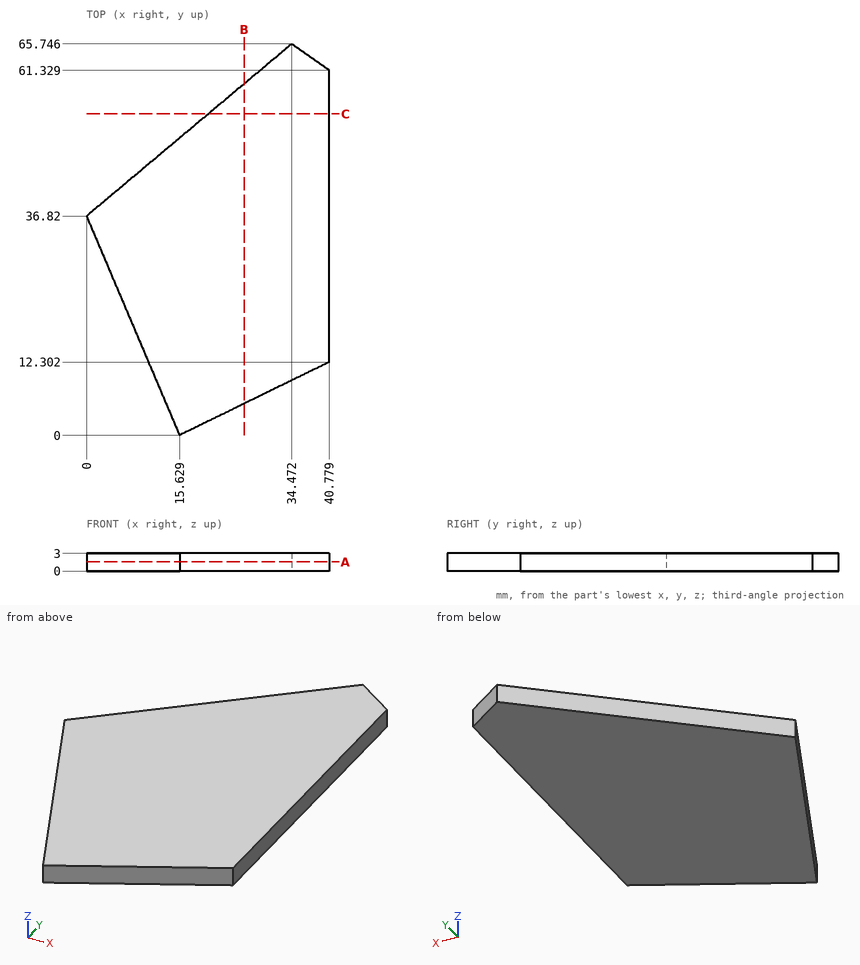
Source: three-view drawing plus pictorial views. Frame: mm from the lowest corner of the part. Round coordinates to 2 decimals unless told otherwise and drop trailing zeros. Loops run counter-clockwise (first coordinate to the right, second up) from the corner with the lowest first, then second, coordinate; pieces in that order, holes last. Notation, with made-up numbers: M -5.5,67.5 L 17.5,67.5 A4 cw 17.5,71.5 Z; hole C 86,73 d6. An arc over 180 degrees is marked long. Put each result on its own line as item: value. Start each with the question number.
(1) Contact query for a flat-ended pin moving along its axis: pin 1 Ø8 at (x, y) = (9.5, 22) entering from -Z. Output: stop coordinate, or through.
(2) Section query A-A (z = 1.55). Return loops of the section in (x, y) (1 decimal), then the cut area to 3 significant figures.
(3) Material intervals for line 1 along X through (y, z) = (27, 0.65); line 2 along Y through (x, z) = (23, 1.5) (1 decimal); line 3 along Y through (x, z) = (9.5, 1.85) (1 decimal), sorted ascending. Write a range as [from, to].
(4) Section query C-C (y = 54). Return loops of the section in (x, z) (1 decimal).
(5) Section query B-B (x = 26.5). Return loops of the section in (y, z), then the cut area to 3 significant figures.
Findings below:
1. pin 1: stops at z = 0
2. outline: M 0,36.8 L 15.6,0 L 40.8,12.3 L 40.8,61.3 L 34.5,65.7 Z
2. area: 1,730 mm2
3. line 1: x = [4.17, 40.78]
3. line 2: y = [3.6, 56.1]
3. line 3: y = [14.4, 44.8]
4. outline: M 20.5,0 L 40.8,0 L 40.8,3 L 20.5,3 Z
5. outline: M 5.32,0 L 59.06,0 L 59.06,3 L 5.32,3 Z
5. area: 161 mm2
